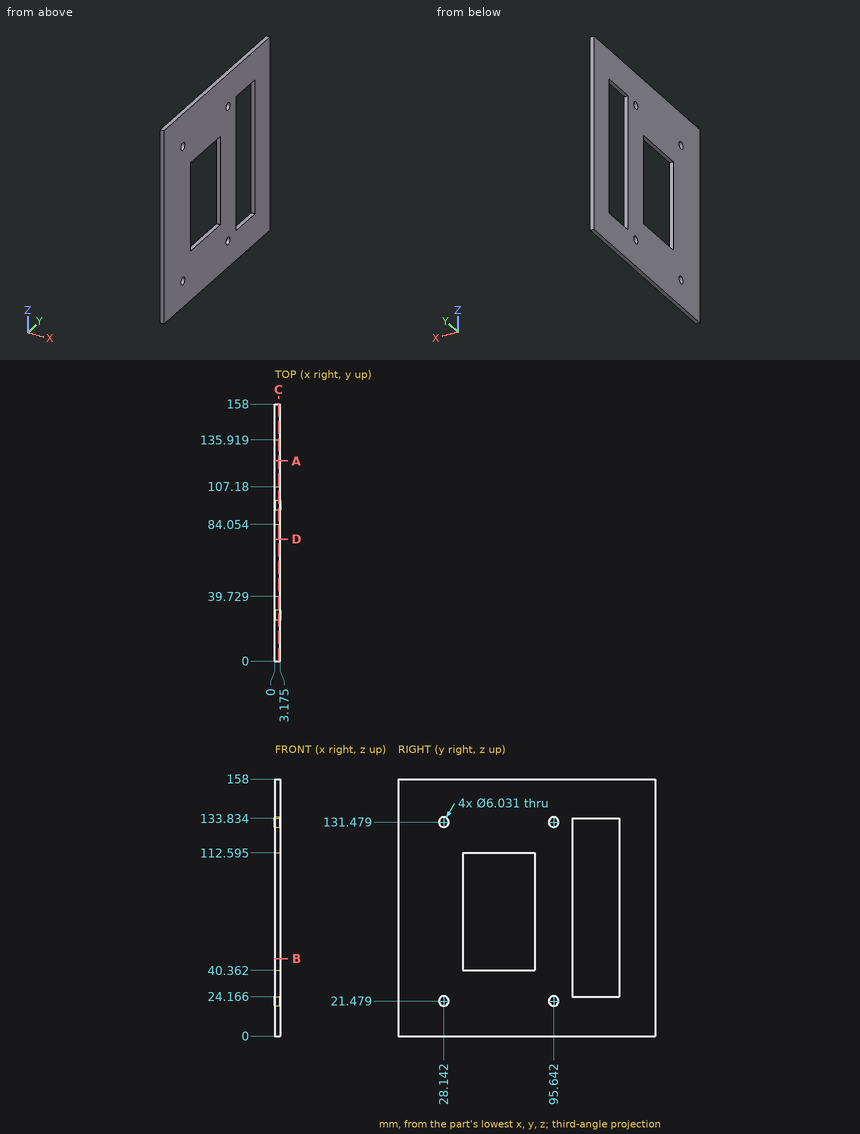
Source: three-view drawing plus pictorial views. Frame: mm from the lowest corner of the part. Coordinates: 2 decimals unless noted, no trailing zeros. Loops run counter-clockwise (first coordinate to the right, second up) from the corner with the lowest first, then second, coordinate; pieces in that order, holes last. Notation, with made-up numbers: (34.5, 28.5) - (56.5, 28.5) arc R17 ccw to (56.5, 46.5) - close; hole circle Ø1 at (71, -10). An arc over 180 degrees is marked (long way). Answer in a Markdown table with one row per item. Add a question column.
Item 1: Section query B-B on z = 47.5. Return the cut outline in (x, y) (1 decimal).
Item 2: Line query: line 1 along Y through (x, z) = (0.15, 90.5) (1 decimal); line 2 along Z through (x, y) = (2.6, 108) (1 decimal); line 3 along Z through (x, y) = (0.55, 82) (1 decimal). Output: solid intervals per line, ascending. Write a range as [from, to].
Item 3: Section query D-D on y = 75. Return the cut outline in (x, z) (1 decimal).
Item 4: Section query A-A on y = 123. Return the cut outline in (x, z) (1 decimal).
Item 5: Section query C-C on x = 2.25. Return the cut outline in (y, z) (1 decimal).
Recorded:
| question | item | result |
|---|---|---|
| 1 | outline | (0, 0) - (3.2, 0) - (3.2, 39.7) - (0, 39.7) - close; (0, 84.1) - (3.2, 84.1) - (3.2, 107.2) - (0, 107.2) - close; (0, 135.9) - (3.2, 135.9) - (3.2, 158) - (0, 158) - close |
| 2 | line 1 | [0, 39.7], [84.1, 107.2], [135.9, 158] |
| 2 | line 2 | [0, 24.2], [133.8, 158] |
| 2 | line 3 | [0, 40.4], [112.6, 158] |
| 3 | outline | (0, 0) - (3.2, 0) - (3.2, 40.4) - (0, 40.4) - close; (0, 112.6) - (3.2, 112.6) - (3.2, 158) - (0, 158) - close |
| 4 | outline | (0, 0) - (3.2, 0) - (3.2, 24.2) - (0, 24.2) - close; (0, 133.8) - (3.2, 133.8) - (3.2, 158) - (0, 158) - close |
| 5 | outline | (0, 0) - (158, 0) - (158, 158) - (0, 158) - close; hole circle Ø6 at (28.1, 21.5); hole circle Ø6 at (28.1, 131.5); hole (39.7, 40.4) - (84.1, 40.4) - (84.1, 112.6) - (39.7, 112.6) - close; hole circle Ø6 at (95.6, 21.5); hole circle Ø6 at (95.6, 131.5); hole (107.2, 24.2) - (135.9, 24.2) - (135.9, 133.8) - (107.2, 133.8) - close |
